Geometry: final body of the model. Coordinates: model frame, mm. Face numbers are marked on the shaded views. A direction names the side the tool comes from. Give positions to 0.01 mm unless a question says otherwise; leave off trailing zeros. Loops run counter-clockwise (first coordinate to the right, second up) from the corner with the lowest first, then second, coordinate; pieces in that order, holes last.
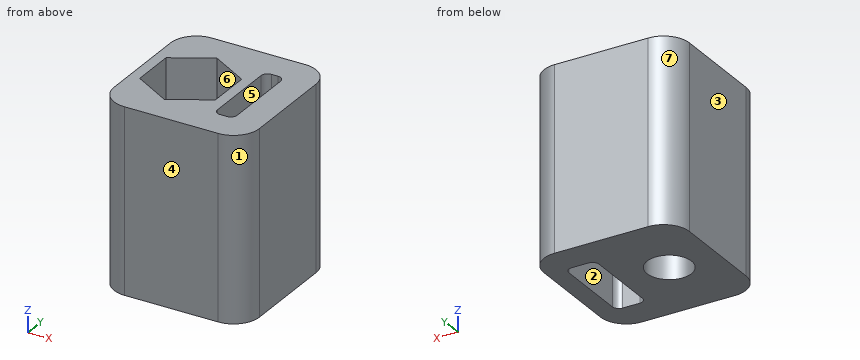
from build123d import *

# Parameters (mm, degrees)
SKETCH1_R           = 1.7
BOSS_EXTRUDE1_DEPTH = 14
CUT_EXTRUDE1_DEPTH  = 4
CUT_EXTRUDE2_DEPTH  = 7


with BuildPart() as part:
    # Sketch1 → Boss-Extrude1 (new body)
    with BuildSketch(Plane.XY):
        with BuildLine():
            Line((-3.695, -3.575), (-3.695, 3.575))
            ThreePointArc((-3.695, 3.575), (-3.116535893, 4.971535893), (-1.72, 5.55))
            Line((-1.72, 5.55), (5.43, 5.55))
            ThreePointArc((5.43, 5.55), (6.826535893, 4.971535893), (7.405, 3.575))
            Line((7.405, 3.575), (7.405, -3.575))
            ThreePointArc((7.405, -3.575), (6.826535893, -4.971535893), (5.43, -5.55))
            Line((5.43, -5.55), (-1.72, -5.55))
            ThreePointArc((-1.72, -5.55), (-3.116535893, -4.971535893), (-3.695, -3.575))
        make_face()
        Circle(SKETCH1_R, mode=Mode.SUBTRACT)
        with BuildLine():
            Line((5.21, 2.75), (5.21, -2.75))
            ThreePointArc((5.21, -2.75), (5.063553391, -3.103553391), (4.71, -3.25))
            Line((4.71, -3.25), (4.21, -3.25))
            ThreePointArc((4.21, -3.25), (3.856446609, -3.103553391), (3.71, -2.75))
            Line((3.71, -2.75), (3.71, 2.75))
            ThreePointArc((3.71, 2.75), (3.856446609, 3.103553391), (4.21, 3.25))
            Line((4.21, 3.25), (4.71, 3.25))
            ThreePointArc((4.71, 3.25), (5.063553391, 3.103553391), (5.21, 2.75))
        make_face(mode=Mode.SUBTRACT)
    extrude(amount=BOSS_EXTRUDE1_DEPTH)

    # Sketch2 → Cut-Extrude1 (cut)
    with BuildSketch(Plane.XY.offset(14)):
        Polygon((0, 3.337084556), (-2.89, 1.668542278), (-2.89, -1.668542278), (0, -3.337084556), (2.89, -1.668542278), (2.89, 1.668542278), align=None)
    extrude(amount=-CUT_EXTRUDE1_DEPTH, mode=Mode.SUBTRACT)

    # Sketch3 → Cut-Extrude2 (cut)
    with BuildSketch(Plane.XY):
        with BuildLine():
            Line((3.71, 2.75), (3.71, -2.75))
            ThreePointArc((3.71, -2.75), (3.856446609, -3.103553391), (4.21, -3.25))
            Line((4.21, -3.25), (5.51, -3.25))
            ThreePointArc((5.51, -3.25), (5.863553391, -3.103553391), (6.01, -2.75))
            Line((6.01, -2.75), (6.01, 2.75))
            ThreePointArc((6.01, 2.75), (5.863553391, 3.103553391), (5.51, 3.25))
            Line((5.51, 3.25), (4.21, 3.25))
            ThreePointArc((4.21, 3.25), (3.856446609, 3.103553391), (3.71, 2.75))
        make_face()
    extrude(amount=CUT_EXTRUDE2_DEPTH, mode=Mode.SUBTRACT)


solid = part.part
Item 1: Section query A-A on y = 0. Return loops of the section in (x, z) (3 decimals), plus the area to 3 significant figures.
Values follow:
outline: (-3.695, 0) - (-1.7, 0) - (-1.7, 10) - (-2.89, 10) - (-2.89, 14) - (-3.695, 14) - close; (1.7, 0) - (3.71, 0) - (3.71, 14) - (2.89, 14) - (2.89, 10) - (1.7, 10) - close; (5.21, 7) - (6.01, 7) - (6.01, 0) - (7.405, 0) - (7.405, 14) - (5.21, 14) - close
area: 71.7 mm2
Item 2: Draft query along X for the marked faces 1, 2, 3 and 4. Return one class per face: +X half, -X half, draft (parallel to the pull), parting line (faces both ways), or undercut.
Values follow:
face 1: +X half
face 2: undercut
face 3: -X half
face 4: draft
Item 3: Pin query (flat end, axial travel): pin 1 (1 mm diameter, centred on y = 4, z = 12, fed in from +X) (3 decimals). Return the tip coordinate at first contact, or that it passes through.
Values follow:
pin 1: stops at x = 7.405
Item 4: Section query D-D on y = -2.5. Return loops of the section in (x, z) (3 decimals), plus the area to 3 significant figures.
Values follow:
outline: (-3.695, 0) - (3.71, 0) - (3.71, 14) - (1.45, 14) - (1.45, 10) - (-1.45, 10) - (-1.45, 14) - (-3.695, 14) - close; (5.21, 7) - (6.01, 7) - (6.01, 0) - (7.405, 0) - (7.405, 14) - (5.21, 14) - close
area: 117 mm2
Item 5: Section query B-B on z = 11. Return loops of the section in (x, y) (3 decimals), plus the area to 3 significant figures.
Values follow:
outline: (-3.695, -3.575) arc R1.975 ccw to (-1.72, -5.55) - (5.43, -5.55) arc R1.975 ccw to (7.405, -3.575) - (7.405, 3.575) arc R1.975 ccw to (5.43, 5.55) - (-1.72, 5.55) arc R1.975 ccw to (-3.695, 3.575) - close; hole (-2.89, -1.669) - (0, -3.337) - (2.89, -1.669) - (2.89, 1.669) - (0, 3.337) - (-2.89, 1.669) - close; hole (3.71, -2.75) arc R0.5 ccw to (4.21, -3.25) - (4.71, -3.25) arc R0.5 ccw to (5.21, -2.75) - (5.21, 2.75) arc R0.5 ccw to (4.71, 3.25) - (4.21, 3.25) arc R0.5 ccw to (3.71, 2.75) - close
area: 81.4 mm2
Item 6: Ray query, probe 1 along X at (y, z) = (0, 3.25) (3 decimals); probe 2 along X at (y, z) = (0, 7.5) (3 decimals); probe 3 along Y at (x, z) = (0, 6.75). Return the intervals inside material, ascending.
Values follow:
probe 1: x = -3.695 to -1.7, 1.7 to 3.71, 6.01 to 7.405
probe 2: x = -3.695 to -1.7, 1.7 to 3.71, 5.21 to 7.405
probe 3: y = -5.55 to -1.7, 1.7 to 5.55
Item 7: Set-up query: the marked faces 5, 6 and 7. Return all of +Z, -Z, +X, -X, +Y, -Y with unobstructed straight access to the full face (end or side cutting, diameter ignored); none if empty.
Values follow:
face 5: +Z, -Z
face 6: +Z
face 7: +Z, -Z, -X, +Y
Item 8: Section query C-C on x = -1.25. Return loops of the section in (y, z), plus the area to 3 significant figures.
Values follow:
outline: (-5.55, 0) - (-1.15, 0) - (-1.15, 10) - (-2.62, 10) - (-2.62, 14) - (-5.55, 14) - close; (1.15, 0) - (5.55, 0) - (5.55, 14) - (2.62, 14) - (2.62, 10) - (1.15, 10) - close
area: 111 mm2
